Check sheet for the modelled part. Datum: model origin and axes. Units: mm. Face numbers are marked on the shaded views. A direction names the side the tool comes from. Round coordinates to 2 decimals unless told otherwise and drop trailing zeros. Loops run counter-clockwise (first coordinate to the right, second up) from the corner with the lowest first, then second, coordinate; pieces in that order, holes last. Notation, with made-up numbers: (79, 13) - (98, 13) arc R36 cw to (98, 48) - close; hole circle Ø8 at (49, 12.25). An arc over 180 degrees is marked (long way). Put each result on its own line as item: value. Start each with the question number.
Item 1: Section check A-A, the plane y = 13. Record the cut outline in (x, z), and give its area (3 significant figures).
Item 2: Section check B-B, the plane x = 74.5. Record the cut outline in (y, z), and give its area (3 significant figures).
Item 3: Section check C-C, the plane z = -35. Record the cut outline in (x, y).
Item 4: Tool access check on the marked faces 1 and 2. Record the directions out of +Z, -Z, +X, -X, +Y, -Y that give a thin tool (end or side, any length) a straight path to the whole face; none if there is none.
Item 5: Gauge pin test, flat ends, axial feed: pin 1 Ø10 at (x, y) = (-31, 9) entering from +Z; pin 2 Ø8.5 at (y, z) = (14.5, 36) entering from +X; pin 3 Ø3.5 at (x, y) = (-52.5, 5) entering from -Z. Record the tip position at first contact, or that the pin passes through.
Item 6: Section check D-D, the plane z = -74.5. Record the cut outline in (x, y), and give its area (3 significant figures).
Item 7: Material ranges on line 1 along X through (y, z) = (1, -90.75); line 2 along Z through (x, y) = (89.75, 3.1); line 3 along X through (y, z) = (4.5, -86.5), recorded low to high.
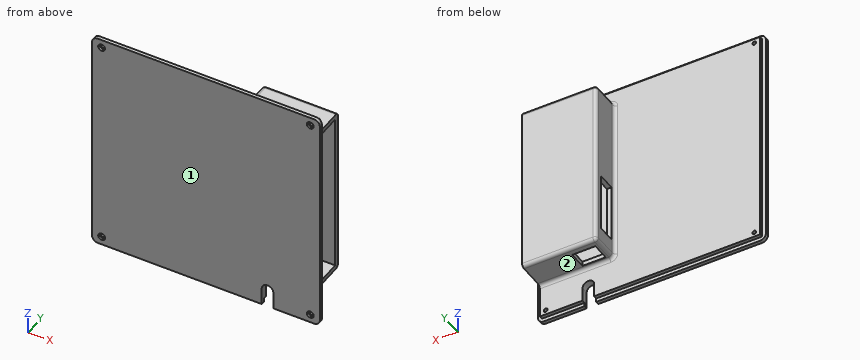
from build123d import *

# Parameters (mm, degrees)
SKETCH1_W               = 196
SKETCH1_H               = 196
BOSS_EXTRUDE1_DEPTH     = 3
FILLET1_R               = 5
SKETCH2_W               = 189.5
SKETCH2_H               = 189.5
BOSS_EXTRUDE2_DEPTH     = 6
SKETCH3_R               = 1.6
CUT_EXTRUDE1_DEPTH      = 139.722745071
SKETCH5_R               = 3
CUT_EXTRUDE5_DEPTH      = 2
MIRROR2_COPY_1_SKETCH_R = 1.6
MIRROR2_COPY_1_DEPTH    = 139.722745071
MIRROR2_COPY_2_SKETCH_R = 3
MIRROR2_COPY_2_DEPTH    = 2
BOSS_EXTRUDE3_DEPTH     = 22
SKETCH7_W               = 64
SKETCH7_H               = 148
BOSS_EXTRUDE4_DEPTH     = 4
FILLET2_R               = 3
CUT_EXTRUDE6_REACH      = 166.938
SKETCH8_W               = 50
SKETCH8_H               = 15
CUT_EXTRUDE7_REACH      = 195.077
SKETCH10_W              = 20
SKETCH10_H              = 15
CUT_EXTRUDE8_DEPTH      = 143.239235094


with BuildPart() as part:
    # Sketch1 → Boss-Extrude1 (new body)
    with BuildSketch(Plane(origin=(0, 0, 0), x_dir=(1, 0, 0), z_dir=(0, 1, 0))):
        Rectangle(SKETCH1_W, SKETCH1_H)
    extrude(amount=BOSS_EXTRUDE1_DEPTH)

    # Fillet1
    fillet1_edges = [part.edges().sort_by_distance(p)[0] for p in [
        (-98, 1.5, -98),
        (-98, 1.5, 98),
        (98, 1.5, 98),
        (98, 1.5, -98),
    ]]
    fillet(fillet1_edges, radius=FILLET1_R)

    # Sketch2 → Boss-Extrude2 (add)
    with BuildSketch(Plane.XZ):
        Rectangle(SKETCH2_W, SKETCH2_H)
    extrude(amount=-BOSS_EXTRUDE2_DEPTH)

    # Sketch3 → Cut-Extrude1 (cut, through all)
    with BuildSketch(Plane(origin=(0, 6, 0), x_dir=(1, 0, 0), z_dir=(0, 1, 0))):
        with Locations(Location((-89.75, 90.75, 0), (0, 0, 270))):
            Circle(SKETCH3_R)
    cut_extrude1 = extrude(amount=-CUT_EXTRUDE1_DEPTH, mode=Mode.SUBTRACT)

    # Sketch5 → Cut-Extrude5 (cut)
    with BuildSketch(Plane.XZ):
        with Locations(Location((-89.75, -90.75, 0), (0, 0, 270))):
            Circle(SKETCH5_R)
    cut_extrude5 = extrude(amount=-CUT_EXTRUDE5_DEPTH, mode=Mode.SUBTRACT)

    # Mirror1: Cut-Extrude1, Cut-Extrude5 across plane
    add(cut_extrude1.mirror(Plane.XY), mode=Mode.SUBTRACT)
    add(cut_extrude5.mirror(Plane.XY), mode=Mode.SUBTRACT)

    # Mirror2: Cut-Extrude1, Cut-Extrude5 across plane
    add(cut_extrude1.mirror(Plane(origin=(0, 0, 0), x_dir=(0, 0, 1), z_dir=(1, 0, 0))), mode=Mode.SUBTRACT)
    add(cut_extrude5.mirror(Plane(origin=(0, 0, 0), x_dir=(0, 0, 1), z_dir=(1, 0, 0))), mode=Mode.SUBTRACT)

    # Mirror2 copy 1 sketch → Mirror2 copy 1 (cut, through all)
    with BuildSketch(Plane(origin=(0, 6, 0), x_dir=(-1, 0, 0), z_dir=(0, 1, 0))):
        with Locations(Location((-89.75, 90.75, 0), (0, 0, 270))):
            Circle(MIRROR2_COPY_1_SKETCH_R)
    extrude(amount=-MIRROR2_COPY_1_DEPTH, mode=Mode.SUBTRACT)

    # Mirror2 copy 2 sketch → Mirror2 copy 2 (cut)
    with BuildSketch(Plane(origin=(0, 0, 0), x_dir=(-1, 0, 0), z_dir=(0, -1, 0))):
        with Locations(Location((-89.75, -90.75, 0), (0, 0, 270))):
            Circle(MIRROR2_COPY_2_SKETCH_R)
    extrude(amount=-MIRROR2_COPY_2_DEPTH, mode=Mode.SUBTRACT)

    # Sketch6 → Boss-Extrude3 (add)
    with BuildSketch(Plane(origin=(0, 6, 0), x_dir=(1, 0, 0), z_dir=(0, 1, 0))):
        Polygon((94.75, -82.75), (94.75, -78.75), (34.75, -78.75), (34.75, 61.25), (94.75, 61.25), (94.75, 65.25), (30.75, 65.25), (30.75, -82.75), align=None)
    extrude(amount=BOSS_EXTRUDE3_DEPTH)

    # Sketch7 → Boss-Extrude4 (add)
    with BuildSketch(Plane(origin=(0, 28, 0), x_dir=(1, 0, 0), z_dir=(0, 1, 0))):
        with Locations((62.75, -8.75)):
            Rectangle(SKETCH7_W, SKETCH7_H)
    extrude(amount=BOSS_EXTRUDE4_DEPTH)

    # Fillet2
    fillet2_edges = [part.edges().sort_by_distance(p)[0] for p in [
        (62.75, 6, 82.75),
        (30.75, 19, 82.75),
        (62.75, 6, -65.25),
        (30.75, 6, 8.75),
        (30.75, 19, -65.25),
        (30.75, 32, 8.75),
        (62.75, 32, 82.75),
        (62.75, 32, -65.25),
    ]]
    fillet(fillet2_edges, radius=FILLET2_R)

    # Sketch8 → Cut-Extrude6 (cut, up to next)
    with BuildSketch(Plane.ZY.offset(-30.75), mode=Mode.PRIVATE) as cut_extrude6_sk1:
        with Locations((-25.25, 17.5)):
            Rectangle(SKETCH8_W, SKETCH8_H)
    cut_extrude6_tool1 = extrude(cut_extrude6_sk1.sketch, amount=-CUT_EXTRUDE6_REACH, mode=Mode.PRIVATE) & part.part
    add(cut_extrude6_tool1.solids().sort_by_distance((30.75, 17.5, -25.25))[0], mode=Mode.SUBTRACT)

    # Sketch10 → Cut-Extrude7 (cut, up to next)
    with BuildSketch(Plane(origin=(0, 0, -65.25), x_dir=(-1, 0, 0), z_dir=(0, 0, -1)), mode=Mode.PRIVATE) as cut_extrude7_sk1:
        with Locations((-45.75, 17.5)):
            Rectangle(SKETCH10_W, SKETCH10_H)
    cut_extrude7_tool1 = extrude(cut_extrude7_sk1.sketch, amount=-CUT_EXTRUDE7_REACH, mode=Mode.PRIVATE) & part.part
    add(cut_extrude7_tool1.solids().sort_by_distance((45.75, 17.5, -65.25))[0], mode=Mode.SUBTRACT)

    # Sketch11 → Cut-Extrude8 (cut, through all)
    with BuildSketch(Plane.XZ):
        with BuildLine():
            Line((58, -98), (48, -98))
            Line((48, -98), (48, -83))
            ThreePointArc((48, -83), (53, -78), (58, -83))
            Line((58, -83), (58, -98))
        make_face()
    extrude(amount=-CUT_EXTRUDE8_DEPTH, mode=Mode.SUBTRACT)


solid = part.part
Check result:
1. outline: (30.75, -62.25) arc R3 ccw to (33.75, -65.25) - (35.75, -65.25) - (35.75, -61.25) - (34.75, -61.25) - (34.75, -50.25) - (30.75, -50.25) - close; (30.75, -0.25) - (34.75, -0.25) - (34.75, 78.75) - (94.75, 78.75) - (94.75, 82.75) - (33.75, 82.75) arc R3 ccw to (30.75, 79.75) - close; (55.75, -65.25) - (94.75, -65.25) - (94.75, -61.25) - (55.75, -61.25) - close
1. area: 788 mm²
2. outline: (0, -98) - (3, -98) - (3, -94.75) - (6, -94.75) - (6, -68.25) arc R3 cw to (9, -65.25) - (29, -65.25) arc R3 ccw to (32, -62.25) - (32, 79.75) arc R3 ccw to (29, 82.75) - (9, 82.75) arc R3 cw to (6, 85.75) - (6, 94.75) - (3, 94.75) - (3, 98) - (0, 98) - close; hole (6, -61.25) - (28, -61.25) - (28, 78.75) - (6, 78.75) - close
2. area: 1,920 mm²
3. outline: (-98, 0) - (98, 0) - (98, 3) - (94.75, 3) - (94.75, 6) - (34.75, 6) - (34.75, 10) - (30.75, 10) - (30.75, 9) arc R3 cw to (27.75, 6) - (-94.75, 6) - (-94.75, 3) - (-98, 3) - close; (30.75, 25) - (34.75, 25) - (34.75, 28) - (94.75, 28) - (94.75, 32) - (33.75, 32) arc R3 ccw to (30.75, 29) - close
4. face 1: +Z, -Z, +X, -X, -Y
4. face 2: -Z, +X, -X, +Y
5. pin 1: z = 94.75
5. pin 2: x = 34.75
5. pin 3: z = -94.75
6. outline: (-98, 0) - (98, 0) - (98, 3) - (94.75, 3) - (94.75, 6) - (-94.75, 6) - (-94.75, 3) - (-98, 3) - close
6. area: 1,160 mm²
7. line 1: -98 to -92.75, -86.75 to 48, 58 to 86.75, 92.75 to 98
7. line 2: -94.75 to -92.35, -89.15 to 89.15, 92.35 to 94.75
7. line 3: -94.75 to 48, 58 to 94.75
